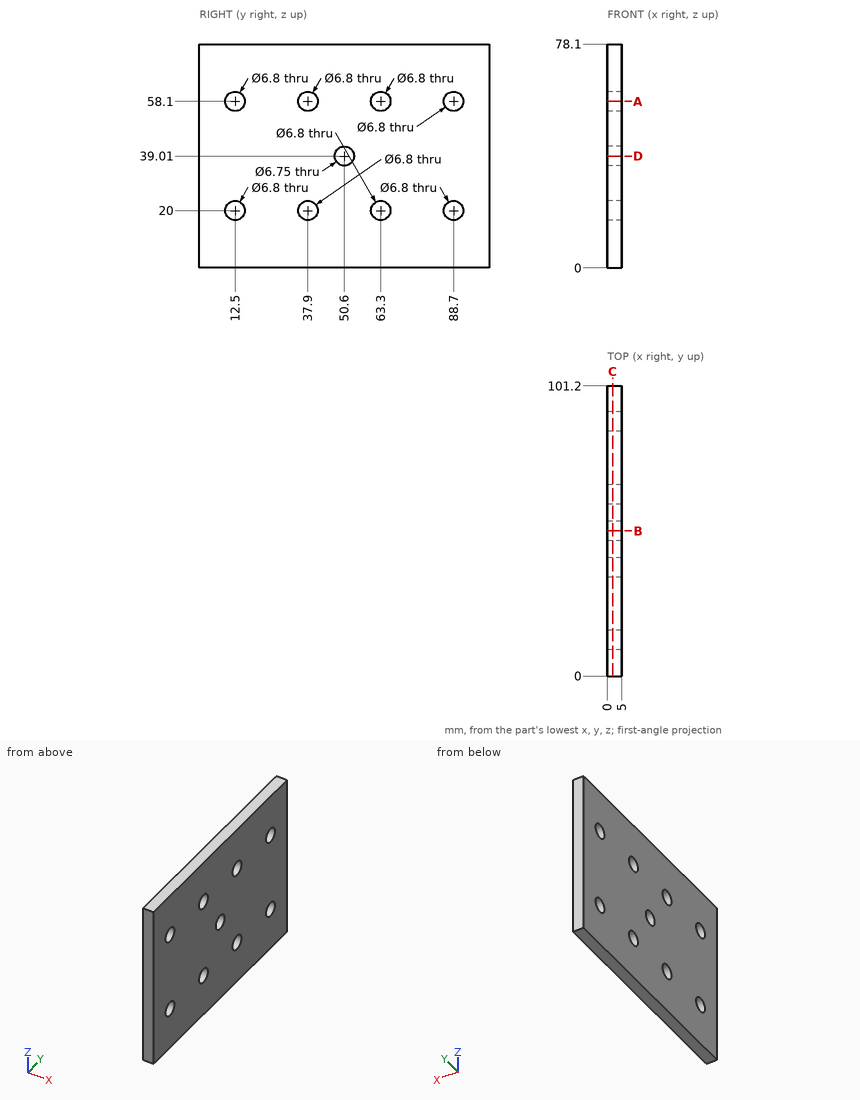
Input: dimensioned drawing with shaded views. Units: mm. Origin: part minimum x, y, z. Round coordinates to 2 decimals unless told otherwise and drop trailing zeros. Loops run counter-clockwise (first coordinate to the right, second up) from the corner with the lowest first, then second, coordinate; pieces in that order, holes last. Notation, with made-up numbers: (-24, -35.75) -> (-13, -35.75) arc R16 ccw to (-13, -19.75) -> close; hole circle Ø11 at (19.25, 51.25). An arc over 180 degrees is marked (long way). Answer as a JSON object with one key per item and string values. Group by question number.
1) Section query D-D on z = 39.01. Output: boundary loops of the cut face in (x, y) (3 decimals), plus the area to 3 significant figures.
2) Section query B-B on y = 50.6. Output: boundary loops of the cut face in (x, z) (3 decimals).
3) Ray query, L1, parallel to Z at x = 3.6, y = 63.3; L2, parallel to Y at x = 2.7, z = 20; L3, parallel to Z at x = 3.95, y = 40. Return the intervals inside material, ascending.
4) Section query A-A on z = 58.1. Output: boundary loops of the cut face in (x, y), plus the area to 3 significant figures.
5) Section query C-C on x = 1.8. State how many separate pieces and enclosed holes the cut face has, plus the area to 3 significant figures.
Reply:
{
 "1": {"outline": "(0, 0) -> (5, 0) -> (5, 47.225) -> (0, 47.225) -> close; (0, 53.975) -> (5, 53.975) -> (5, 101.2) -> (0, 101.2) -> close", "area": "472 mm2"},
 "2": {"outline": "(0, 0) -> (5, 0) -> (5, 35.635) -> (0, 35.635) -> close; (0, 42.385) -> (5, 42.385) -> (5, 78.1) -> (0, 78.1) -> close"},
 "3": {"L1": "z = 0 to 16.6, 23.4 to 54.7, 61.5 to 78.1", "L2": "y = 0 to 9.1, 15.9 to 34.5, 41.3 to 59.9, 66.7 to 85.3, 92.1 to 101.2", "L3": "z = 0 to 17.33, 22.67 to 55.43, 60.77 to 78.1"},
 "4": {"outline": "(0, 0) -> (5, 0) -> (5, 9.1) -> (0, 9.1) -> close; (0, 15.9) -> (5, 15.9) -> (5, 34.5) -> (0, 34.5) -> close; (0, 41.3) -> (5, 41.3) -> (5, 59.9) -> (0, 59.9) -> close; (0, 66.7) -> (5, 66.7) -> (5, 85.3) -> (0, 85.3) -> close; (0, 92.1) -> (5, 92.1) -> (5, 101.2) -> (0, 101.2) -> close", "area": "370 mm2"},
 "5": {"separate pieces": "1", "enclosed holes": "9", "area": "7,580 mm2"}
}
